```python
from build123d import *

# Parameters (mm, degrees)
F0_R   = 6
F0_R_2 = 5


with BuildPart() as f3:
    # F3: sweep along a path in F2
    with BuildLine(Plane(origin=(0, 0, 0), x_dir=(0, -1, 0), z_dir=(-0.989728, 0, 0.142961))) as f3_path:
        Line((0, 0), (-107.95, 0))
        ThreePointArc((-107.95, 0), (-116.930256, -3.719744), (-120.65, -12.7))
        Line((-120.65, -12.7), (-120.65, -102.786233))
        ThreePointArc((-120.65, -102.786233), (-116.930256, -111.766489), (-107.95, -115.486233))
        Line((-107.95, -115.486233), (-98.428674, -115.486233))
    # F0 (on Front) → F3 (sweep)
    with BuildSketch(Plane.XZ):
        Circle(F0_R)
        Circle(F0_R_2, mode=Mode.SUBTRACT)
    sweep(path=f3_path.line)


solid = f3.part
```
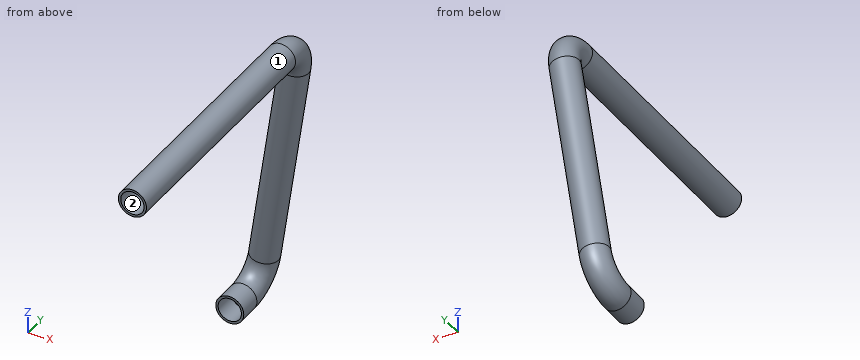
Can you work these out from the model? Positions are in its coordinate system, mm. Face numbers are marked on the shaded views. Give positions to 0.01 mm unless a question says otherwise; leave off trailing zeros. Order: outer loops, then holes, each group sorted by start corner. A loop starts at its lowest first (then second) coordinate and runs counter-clockwise, first axis right, second up. Notation, with made-up numbers: (61, -38.75) - (108, -38.75) arc R17 ccw to (108, -28.75) - close; hole circle Ø8 at (55, 39). An arc over 180 degrees is marked (long way). Use a Markdown table: item, result. Add a question column.
Q1. Please list where these lines run through material, in increasing order: line 1 along Y through (x, z) = (-2, -14.5); line 2 along Z through (x, y) = (0, 53); line 3 along Z through (x, y) = (-12.25, 108).
Q2. If we mould it in two halves opening along X, with no side actions, what happens to the marked faces 1 and 2? For each: released by +X, released by -X, zero draft, split by the parting line, or undercut.
Q3. If we section it at A-A on y = 17: Write out the boundary of the cut face in (x, z), plus the area to 3 significant figures.
Q4. If we section it at B-B on y = 110: Count the separate pieces of the cut face and the enclosed holes in it, plus the area to 3 significant figures.
Q5. I'm going to push flat-ended pins straight in: pin 1 (8 mm diameter, centred on x = -1.5, z = -44, fed in from +Y); pin 2 (3.5 mm diameter, centred on x = -14, z = -117, fed in from -Y); pin 3 (4 mm diameter, centred on x = -8, z = -83.5, fed in from -Y). Where does each tip first touch, or does it pass through?
Answers follow:
| question | item | result |
|---|---|---|
| 1 | line 1 | y = 114.65 to 115.65, 125.65 to 126.65 |
| 1 | line 2 | z = -6 to -5, 5 to 6 |
| 1 | line 3 | z = -118.53 to -116.92, -111.68 to -110.07 |
| 2 | face 1 | split by the parting line |
| 2 | face 2 | undercut |
| 3 | outline | circle Ø12 at (0, 0); hole circle Ø10 at (0, 0) |
| 3 | area | 34.6 mm^2 |
| 4 | separate pieces | 2 |
| 4 | enclosed holes | 2 |
| 4 | area | 70.4 mm^2 |
| 5 | pin 1 | stops at y = 126.6 |
| 5 | pin 2 | stops at y = 98.43 |
| 5 | pin 3 | stops at y = 115 |
